Verification items for the finished model (mm, model axes). A direction names the side the tool comes from. Give positions to 0.01 mm unless a question says otherwise; leave off trailing zeros. Write each loop counter-clockwise with the first axis right and the second up, starting at its lowest first coordinate (ties: lowest second). Pieces come first, ordered by that corner, then holes. Notation, with made-up numbers: M 64.5,61 L 122.5,61 A15 ccw 122.5,80 Z; hole C -18,80 d7. An arc over 180 degrees is marked long. Write item = value, one per line.
from build123d import *

# Parameters (mm, degrees)
SKETCH1_R           = 0.75
BOSS_EXTRUDE1_DEPTH = 2


with BuildPart() as part:
    # Sketch1 → Boss-Extrude1 (new body)
    with BuildSketch(Plane.XY):
        with BuildLine():
            Line((4.948803726, 2), (-1.5, 2))
            ThreePointArc((-1.5, 2), (-2.207106781, 1.707106781), (-2.5, 1))
            Line((-2.5, 1), (-2.5, -6))
            Line((-2.5, -6), (8.03164583, -6))
            ThreePointArc((8.03164583, -6), (10.136786902, -5.885360204), (12.217030025, -5.542796686))
            ThreePointArc((12.217030025, -5.542796686), (14.533048705, -0.947048427), (9.566127614, 0.4))
            Line((9.566127614, 0.4), (7.566127614, 0.4))
            ThreePointArc((7.566127614, 0.4), (7.005701644, 0.571795477), (6.637832967, 1.028154536))
            ThreePointArc((6.637832967, 1.028154536), (6.20529876, 1.623025524), (5.541978268, 1.940772681))
            ThreePointArc((5.541978268, 1.940772681), (5.246865763, 1.985156448), (4.948803726, 2))
        make_face()
        Circle(SKETCH1_R, mode=Mode.SUBTRACT)
        with Locations((5, 0)):
            Circle(SKETCH1_R, mode=Mode.SUBTRACT)
    extrude(amount=BOSS_EXTRUDE1_DEPTH)


solid = part.part
1) Material ranges on probe 1 along Y at (x, z) = (5, 1); probe 2 along Y at (x, z) = (8.25, 0.4); probe 3 along X at (y, z) = (-0.5, 0.45), recorded low to high. Write a range as from..to.
From the geometry:
probe_1 = -6..-0.75, 0.75..2
probe_2 = -6..0.4
probe_3 = -2.5..-0.56, 0.56..4.44, 5.56..14.29
2) Cross-section at C-C on x = 11.5. Record the boundary of the cut face in (y, z), plus the area to 3 significant figures.
From the geometry:
outline = M -5.69,0 L 1.02,0 L 1.02,2 L -5.69,2 Z
area = 13.4 mm^2
3) Cross-section at B-B on z = 0.25. Record the boundary of the cut face in (x, y), plus the area to 3 significant figures.
From the geometry:
outline = M -2.5,-6 L 8.03,-6 A19.39 ccw 12.22,-5.54 A3.32 ccw long 9.57,0.4 L 7.57,0.4 A1 cw 6.64,1.03 A1.5 ccw 5.54,1.94 A3 ccw 4.95,2 L -1.5,2 A1 ccw -2.5,1 Z; hole C 0,0 d1.5; hole C 5,0 d1.5
area = 118 mm^2
4) Draft check along X on faces 3 (the flat face through (3, -6, 1)), 4 (the cylindrical face through (6.21, 1.62, 0.99)), 5 (the cylindrical face through (14.566, -1.023, 0.986)). Enter one of: +X half, -X half, draft (parallel to the pull), parting line (faces both ways), or undercut.
From the geometry:
face_3 = draft
face_4 = +X half
face_5 = undercut
5) Tool access check on faces 1 (the flat face through (-2.5, -2, 1)), 2 (the cylindrical face through (7.01, 0.57, 0.99)). Record the directions out of +Z, -Z, +X, -X, +Y, -Y that give a thin tool (end or side, any length) a straight path to the whole face; none if there is none.
From the geometry:
face_1 = +Z, -Z, -X, +Y, -Y
face_2 = +Z, -Z, +Y
6) Cross-section at D-D on y = 1.5. Record the boundary of the cut face in (x, z), plus the area to 3 significant figures.
From the geometry:
outline = M -2.37,0 L 6.34,0 L 6.34,2 L -2.37,2 Z
area = 17.4 mm^2
7) Depth check by flat-ended pin: P1, Ø1, axis at y = -1, z = 2, coming from the +X side; P2, Ø0.9, axis at x = 5, y = 0, coming from the -Z side. Enter the tip coordinate at first touch or a pass-through.
From the geometry:
P1 = 14.72
P2 = through
8) Cross-section at A-A on y = -0.5. Record the boundary of the cut face in (x, z).
From the geometry:
outline = M -2.5,0 L -0.56,0 L -0.56,2 L -2.5,2 Z; M 0.56,0 L 4.44,0 L 4.44,2 L 0.56,2 Z; M 5.56,0 L 14.29,0 L 14.29,2 L 5.56,2 Z
